Here's how the part is built. I have some questions about the finished solid (model axes, mm). A direction names the side the tool comes from. Coordinates: 2 decimals unless noted, no trailing zeros. Order: outer loops, then holes, each group sorted by start corner. A loop starts at its lowest first (then second) coordinate and runs counter-clockwise, first axis right, second up. Notation, with made-up numbers: (43, 62) - (95, 62) arc R30 ccw to (95, 100) - close; hole circle Ø2 at (54, 80.25). An arc over 180 degrees is marked (long way). Answer as CSV lines item,"result". Start each with the question number.
Q1. Suppose I cut it at C-C (z = 0.5). Please give me the cut outline in (x, y), then the cut area to 3 significant figures.
Q2. For faces 4 (the face through (1.11, 5.02, -1)), 5 (the face through (-0.4, -3.02, 2.84)), 6 (the face through (-5.5, 0.2, -2.032)), which set-ups out of +Z, -Z, +X, -X, +Y, -Y let a thin tool reach every point of the face, with its end or its side?
Q3. For pin 1 Ø1 at (x, y) = (7, -4) entering from +Z; pin 2 Ø1.5 at (x, z) = (-9, -1) entering from -Y; pin 3 Ø5 at (x, y) = (-2.5, 0) entering from -Z, each with a flat end and sliding along its axis, tell me the tip position at first contact or that it passes through.
Q4. Suppose I cut it at D-D (x = -7.25). Please give me the cut outline in (y, z), then the cut area to 3 significant figures.
Q5. Suppose I cut it at A-A (x = 0). Please give me the cut outline in (y, z) (1 decimal), then the cut area to 3 significant figures.
Q6. Thinking about a two-plate mould opening in Y: for faces 1 (the face through (5, 0, 1.588)), 2 (the face through (-0.96, 4.34, 2.84)), 3 (the face through (1.1, -1.1, 0)), which applies, released by +Y, released by -Y, zero draft, split by the parting line, or undercut?
Q7. I need wall thicknesses on line 1 (Y direction, x = 0, z = 2.3) (3 decimals); line 2 (Y direction, x = 0, z = -1.25); line 3 (Z direction, x = -2.25, y = -6.75). Which ranges of each line are inside material? Lowest first, please.
Autodesk Inventor part; units mm, degrees
ref_plane "YZ Plane" through (0, 0, 0) normal (1, 0, 0) x (0, 1, 0)
ref_plane "XZ Plane" through (0, 0, 0) normal (0, 1, 0) x (-1, 0, 0)
ref_plane "XY Plane" through (0, 0, 0) normal (0, 0, 1) x (1, 0, 0)
sketch "Sketch1" plane through (0, 0, 0) normal (0, 0, 1) x (1, 0, 0)
  circle A0 centre (0, 0) radius 12.7
  circle A1 centre (0, 0) radius 1.397
  dimension "d0" = 25.4
  dimension "d1" = 2.794
extrude "Extrusion1" add sketch "Sketch1" along normal blind 1.5875
sketch "Sketch2" plane through (0, 0, 1.5875) normal (0, 0, 1) x (1, 0, 0)
  circle A0 centre (0, 0) radius 3.048
  circle A1 centre (0, 0) radius 4.445
  dimension "d4" = 6.096
  dimension "d5" = 8.89
extrude "Extrusion2" add sketch "Sketch2" along normal blind 2.54
sketch "Sketch3" plane through (0, 0, 0) normal (0, 0, -1) x (-1, 0, 0)
  circle A0 centre (0, 0) radius 12.7
  circle A1 centre (0, 0) radius 5.1432
  dimension "d8" = 25.4
extrude "Extrusion3" add sketch "Sketch3" along normal blind 2.032
equation "\"d0\" = hornD"
equation "\"d1\" = hornS"
equation "\"d2\" = hornT"
equation "\"d4\" = hornID"
equation "\"d5\" = hornOD"
equation "\"d6\" = hornH"
equation "\"d8\" = spoolD"
equation "\"d9\" = inset"
equation "\"spoolD\" = 25.4"
equation "\"hubD\" = 6.35"
equation "\"spoolT\" = 1.5875"
equation "\"hubH\" = 6.35"
equation "\"hornD\" = 25.4"
equation "\"hornT\" = 1.5875"
equation "\"hornS\" = 2.794"
equation "\"hornID\" = 6.096"
equation "\"hornOD\" = 8.89"
equation "\"hornH\" = 2.54"
equation "\"inset\" = 2.032"
equation "\"insetD\" = 5.842"
equation "\"servMD\" = 3.175"
equation "\"servMW\" = 10.033"
equation "\"servML\" = 49.784"
equation "\"servW\" = 20.1168"
equation "\"servL\" = 40.5892"
equation "\"housL\" = 53.975"
equation "\"housW\" = 28.575"
equation "\"housT\" = 2.54"
equation "\"housBT\" = 1.5875"
equation "\"housH\" = 39.116"
equation "\"guideW\" = 9.144"
equation "\"guideD\" = 3.175"
equation "\"guideH\" = 23.114"
properties part number "Horn"
Here are the results:
1,outline,"circle Ø25.4 at (0, 0); hole circle Ø2.79 at (0, 0)"
1,area,"501 mm²"
2,face 4,"-Z"
2,face 5,"+Z"
2,face 6,"-Z, +X, -X, +Y, -Y"
3,pin 1,"stops at z = 1.59"
3,pin 2,"stops at y = -9.66"
3,pin 3,"stops at z = 0"
4,outline,"(-10.43, -2.03) - (10.43, -2.03) - (10.43, 1.59) - (-10.43, 1.59) - close"
4,area,"75.5 mm²"
5,outline,"(-12.7, -2) - (-5.1, -2) - (-5.1, 0) - (-1.4, 0) - (-1.4, 1.6) - (-3, 1.6) - (-3, 4.1) - (-4.4, 4.1) - (-4.4, 1.6) - (-12.7, 1.6) - close; (1.4, 0) - (5.1, 0) - (5.1, -2) - (12.7, -2) - (12.7, 1.6) - (4.4, 1.6) - (4.4, 4.1) - (3, 4.1) - (3, 1.6) - (1.4, 1.6) - close"
5,area,"73.7 mm²"
6,face 1,"zero draft"
6,face 2,"split by the parting line"
6,face 3,"undercut"
7,line 1,"y = -4.445 to -3.048, 3.048 to 4.445"
7,line 2,"y = -12.7 to -5.14, 5.14 to 12.7"
7,line 3,"z = -2.03 to 1.59"
